Part model, mm, in its own coordinate system. Face numbers are marked on the shaded views. A direction names the side the tool comes from. Coordinates: 2 decimals unless noted, no trailing zeros. Write each loop counter-clockwise with the first axis right and the second up, starting at its lowest first coordinate (ties: lowest second). Pieces come first, ordered by that corner, then holes. Notation, with made-up numbers: (70.25, -24.5) - (75.25, -24.5) arc R25 cw to (75.25, 6.5) - close; hole circle Ø9 at (-22, -13.75). An arc over 180 degrees is marked (long way). Use a Markdown table: item, result.
```python
from build123d import *

# Parameters (mm, degrees)
CROQUIS1_R              = 10
SALIENTE_EXTRUIR1_DEPTH = 12


with BuildPart() as part:
    # Croquis1 → Saliente-Extruir1 (new body)
    with BuildSketch(Plane.XY):
        with BuildLine():
            Line((0, 0), (0, 70))
            Line((0, 70), (11, 70))
            Line((11, 70), (11, 64.196152423))
            ThreePointArc((11, 64.196152423), (8.204445042, 57.447085729), (14, 53))
            Line((14, 53), (48.5, 53))
            ThreePointArc((48.5, 53), (54.295554958, 57.447085729), (51.5, 64.196152423))
            Line((51.5, 64.196152423), (51.5, 70))
            Line((51.5, 70), (98.5, 70))
            Line((98.5, 70), (98.5, 64.196152423))
            ThreePointArc((98.5, 64.196152423), (95.704445042, 57.447085729), (101.5, 53))
            Line((101.5, 53), (136, 53))
            ThreePointArc((136, 53), (141.795554958, 57.447085729), (139, 64.196152423))
            Line((139, 64.196152423), (139, 70))
            Line((139, 70), (150, 70))
            Line((150, 70), (150, 0))
            Line((150, 0), (0, 0))
        make_face()
        with Locations((75, 53)):
            Circle(CROQUIS1_R, mode=Mode.SUBTRACT)
    extrude(amount=SALIENTE_EXTRUIR1_DEPTH)


solid = part.part
```
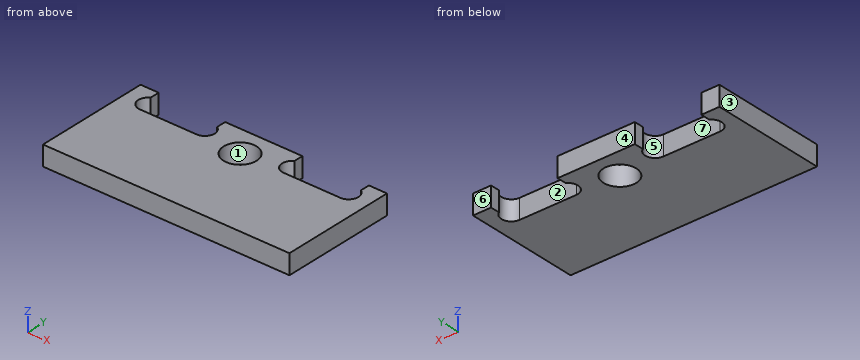
Item 1: Two-plate mould, pull along X, no slides. Class the marked faces 1, 2, 3 and 4: pulls with the +X half, pulls with the -X half, needs draft (parallel to the pull), parting line crosses it, or undercut.
From the geometry:
| item | result |
|---|---|
| face 1 | undercut |
| face 2 | undercut |
| face 3 | pulls with the -X half |
| face 4 | needs draft |
Item 2: Band-saw the part on D-D, the plane y = 55. Give the cut face in (x, z).
From the geometry:
| item | result |
|---|---|
| outline | (0, 0) - (9.53, 0) - (9.53, 12) - (0, 12) - close; (52.97, 0) - (65.2, 0) - (65.2, 12) - (52.97, 12) - close; (84.8, 0) - (97.03, 0) - (97.03, 12) - (84.8, 12) - close; (140.47, 0) - (150, 0) - (150, 12) - (140.47, 12) - close |
Item 3: Which spindle directions (+Z, -Z, +X, -X, +Y, -Y) get a long thin tool onto all of the face, cutting with end or side? Do the marked faces 5, 6 and 7. Say none if no direction does.
From the geometry:
| item | result |
|---|---|
| face 5 | +Z, -Z |
| face 6 | +Z, -Z, +X, -X, +Y |
| face 7 | +Z, -Z, +Y |
Item 4: Drop a flat-ended pin along its axis: P1, Ø2, axis at x = 18.5, z = 2, coming from the +Y side. Give the stop position or say it passes through.
From the geometry:
| item | result |
|---|---|
| P1 | y = 53 |
Item 5: Band-saw the part on A-A, the plane y = 45. Give the cut face in (x, z).
From the geometry:
| item | result |
|---|---|
| outline | (0, 0) - (69, 0) - (69, 12) - (0, 12) - close; (81, 0) - (150, 0) - (150, 12) - (81, 12) - close |
Item 6: Drill centre lines: probe 1 along Y at (x, z) = (75, 8); probe 2 along X at (y, z) = (52.5, 4); probe 3 along X at (y, z) = (59, 7). Where is each one in solid material? Low to high.
From the geometry:
| item | result |
|---|---|
| probe 1 | 0 to 43, 63 to 70 |
| probe 2 | 0 to 65.01, 84.99 to 150 |
| probe 3 | 0 to 8, 54.5 to 67, 83 to 95.5, 142 to 150 |
Item 7: Band-saw the part on B-B, the plane x = 75. Give the cut face in (y, z), then the cut area to 3 significant figures.
From the geometry:
| item | result |
|---|---|
| outline | (0, 0) - (43, 0) - (43, 12) - (0, 12) - close; (63, 0) - (70, 0) - (70, 12) - (63, 12) - close |
| area | 600 mm^2 |
Item 8: Band-saw the part on C-C, the plane z = 9. Give the cut face in (x, y), then the cut area to 3 significant figures.
From the geometry:
| item | result |
|---|---|
| outline | (0, 0) - (150, 0) - (150, 70) - (139, 70) - (139, 64.2) arc R6 cw to (136, 53) - (101.5, 53) arc R6 cw to (98.5, 64.2) - (98.5, 70) - (51.5, 70) - (51.5, 64.2) arc R6 cw to (48.5, 53) - (14, 53) arc R6 cw to (11, 64.2) - (11, 70) - (0, 70) - close; hole circle Ø20 at (75, 53) |
| area | 8,720 mm^2 |
